from build123d import *

# Parameters (mm, degrees)
BOSS_EXTRU_1_DEPTH   = 15
CONG_1_R             = 3
CONG_2_R             = 4
ESQUISSE2_W          = 22
ESQUISSE2_H          = 4
BOSS_EXTRU_2_DEPTH   = 5
D_GAGEMENT_M41_D     = 4.5
D_GAGEMENT_M41_DEPTH = 16


with BuildPart() as part:
    # Esquisse1 → Boss.-Extru.1 (new body)
    with BuildSketch(Plane.XY):
        Polygon((0, 0), (-22, 0), (-22, 4), (-69, 4), (-69, 8), (-56.26016699, 15.95016153), (-56.26016699, 21.33814045), (-64, 25), (-164, 32), (-168, 35), (-168, 43), (-164, 43), (-164, 38), (-74, 38), (-74, 43), (-69, 43), (-45.444881322, 38.157051099), (-25.711083844, 24.413870713), (-13, 4), (0, 4), align=None)
    extrude(amount=BOSS_EXTRU_1_DEPTH)

    # Congé1
    cong_1_edges = [part.edges().sort_by_distance(p)[0] for p in [
        (-119, 38, 0),
        (-119, 38, 15),
    ]]
    fillet(cong_1_edges, radius=CONG_1_R)

    # Congé2
    cong_2_edges = [part.edges().sort_by_distance(p)[0] for p in [
        (-69, 8, 7.5),
        (-164, 32, 7.5),
        (-168, 35, 7.5),
        (-168, 43, 7.5),
        (-69, 43, 7.5),
        (-45.444881322, 38.157051099, 7.5),
        (-25.711083844, 24.413870713, 7.5),
        (-13, 4, 7.5),
    ]]
    fillet(cong_2_edges, radius=CONG_2_R - 0.0001)  # a hair under: the kernel refuses the full size

    # Esquisse2 → Boss.-Extru.2 (add)
    with BuildSketch(Plane(origin=(0, 0, 0), x_dir=(-1, 0, 0), z_dir=(0, 0, -1))):
        with Locations((11, 2)):
            Rectangle(ESQUISSE2_W, ESQUISSE2_H)
    extrude(amount=BOSS_EXTRU_2_DEPTH)

    # Dégagement M41
    with Locations(Plane(origin=(0, 4, 0), x_dir=(1, 0, 0), z_dir=(0, 1, 0))):
        with Locations((-6.5, -5)):
            Hole(D_GAGEMENT_M41_D / 2, depth=D_GAGEMENT_M41_DEPTH)


solid = part.part
For this review, take the finished solid that the model builds, in its own axes (mm). A direction names the side the tool comes from. Give positions to 0.01 mm unless a question says otherwise; leave off trailing zeros. Loops run counter-clockwise (first coordinate to the right, second up) from the corner with the lowest first, then second, coordinate; pieces in that order, holes last.
Item 1: Tool access review of faces 1 (the flat face through (-60.076, 23.143, 7.395)), 2 (the cylindrical face through (-118.37, 37.14, 0.9)), 3 (the flat face through (-45, 4, 7)), 4 (the flat face through (-35.707, 31.375, 7.395)): name each direction out of +Z, -Z, +X, -X, +Y, -Y from which nothing blocks a thin tool from reaching the whole face with its end or side.
Item 2: Take a section at A-A, the plane x = -6.5. State the section outline as (y, z) points, and give its area (3 significant figures).
Item 3: For line 1 along Z through (x, y) = (-6.5, 2.25); line 2 along Z through (x, y) = (-48, 31); line 3 along Y through (x, z) = (-10.5, 9.5), list the stretches that pass through material, from the lowest coordinate up.
Item 4: Insertion check: pin 1 (2.5 mm diameter, centred on x = -137.5, z = 6.5, fed in from +Y); pin 2 (12 mm diameter, centred on x = -49, z = 4, fed in from +Y); pin 3 (4 mm diameter, centred on y = 37.5, z = 4, fed in from +X). Each pin has a flat end and moves straight along its axis. Give the tip position at first contact, or say it passes through.
Item 5: Draft analysis for pull direction Y (two halves, no side actions). For faces 5 (the flat face through (-56.26, 19, 7)), 6 (the flat face through (-57.58, 40.65, 7.4)), 7 (the flat face through (-164, 40, 7)), 8 (the cylindrical face through (-68.51, 7.7, 7.6)), state which applies: +Y half, -Y half, draft (parallel to the pull), parting line (faces both ways), or undercut.
Item 6: Take a section at C-C, the plane x = -154. State the section outline as (y, z) points, and give its area (3 significant figures).
Item 7: Take a section at D-D, the plane x = -62. State the section outline as (y, z) points, and give its area (3 significant figures).
Calculated:
1. face 1: +Z, -Z, -X
1. face 2: -Z, +Y
1. face 3: +Z, -Z, -X, -Y
1. face 4: +Z, -Z, +X, +Y
2. outline: (0, -5) - (4, -5) - (4, 2.75) - (0, 2.75) - close; (0, 7.25) - (4, 7.25) - (4, 15) - (0, 15) - close
2. area: 62.0 mm2
3. line 1: z = -5 to 2.75, 7.25 to 15
3. line 2: z = 0 to 15
3. line 3: y = 0 to 4
4. pin 1: stops at y = 38
4. pin 2: stops at y = 40.12
4. pin 3: stops at x = -41.63
5. face 5: undercut
5. face 6: +Y half
5. face 7: draft
5. face 8: undercut
6. outline: (31.3, 0) - (35, 0) arc R3 ccw to (38, 3) - (38, 12) arc R3 ccw to (35, 15) - (31.3, 15) - close
6. area: 96.6 mm2
7. outline: (4, 0) - (12.37, 0) - (12.37, 15) - (4, 15) - close; (24.05, 0) - (41.56, 0) - (41.56, 15) - (24.05, 15) - close
7. area: 388 mm2
